Source: CAD feature listing. Evaluate the final solid. Frame: model axes, mm. A direction names the side the tool comes from. Give positions to 0.01 mm unless a question says otherwise; leave off trailing zeros. Order: outer loops, then holes, each group sorted by start corner. A loop starts at its lowest first (then second) coordinate and runs counter-clockwise, first axis right, second up. Notation, with made-up numbers: M 37.5,28 L 67.5,28 A27 cw 67.5,67 Z; hole C 59.25,26 d5. An arc over 180 degrees is marked long. Return JSON: item names as keys, results as strings.
from build123d import *

# Parameters (mm, degrees)
SKETCH1_R               = 10
BOSS_EXTRUDE1_DEPTH     = 3
SKETCH2_R               = 6
BOSS_EXTRUDE2_DEPTH     = 5
TAP_DRILL_FOR_M6_TAP1_D = 5


with BuildPart() as part:
    # Sketch1 → Boss-Extrude1 (new body)
    with BuildSketch(Plane.XY):
        Circle(SKETCH1_R)
    extrude(amount=BOSS_EXTRUDE1_DEPTH)

    # Sketch2 → Boss-Extrude2 (add)
    with BuildSketch(Plane(origin=(0, 0, 0), x_dir=(-1, 0, 0), z_dir=(0, 0, -1))):
        Circle(SKETCH2_R)
    extrude(amount=BOSS_EXTRUDE2_DEPTH)

    # Tap Drill for M6 Tap1 (through all)
    with Locations(Plane(origin=(0, 0, -5), x_dir=(-1, 0, 0), z_dir=(0, 0, -1))):
        with Locations((0, 0)):
            Hole(TAP_DRILL_FOR_M6_TAP1_D / 2)


solid = part.part
1. First-contact query: pin 1 (2 mm diameter, centred on x = 6.5, z = 1, fed in from -Y); pin 2 (2 mm diameter, centred on x = 2, z = 0, fed in from +Y); pin 3 (3 mm diameter, centred on x = 6.5, z = -0.5, fed in from +Y). Flat tips, straight axial feed; report the tip coordinate or a pass-through.
Evaluation:
{"pin 1": "stops at y = -8.35", "pin 2": "stops at y = 9.95", "pin 3": "stops at y = 8.61"}
2. Ray query, probe 1 along Y at (x, z) = (0, -2.5); probe 2 along Z at (x, y) = (7.25, -3.25); probe 3 along Y at (x, z) = (0, 2). Return the intervals inside material, ascending.
Evaluation:
{"probe 1": "y = -6 to -2.5, 2.5 to 6", "probe 2": "z = 0 to 3", "probe 3": "y = -10 to -2.5, 2.5 to 10"}
3. Set-up query: faces 1 (the face through (2, -2, 3)), 2 (the face through (6, 0, -2)). Return all of +Z, -Z, +X, -X, +Y, -Y with unobstructed straight access to the full face (end or side cutting, diameter ignored); none if empty.
Evaluation:
{"face 1": "+Z, +X, -X, +Y, -Y", "face 2": "-Z"}
4. Section query A-A (x = 0). Return loops of the section in (y, z), then the cut area to 3 significant figures.
Evaluation:
{"outline": "M -10,0 L -6,0 L -6,-5 L -2.5,-5 L -2.5,3 L -10,3 Z; M 2.5,-5 L 6,-5 L 6,0 L 10,0 L 10,3 L 2.5,3 Z", "area": "80.0 mm^2"}
5. Draft query along X for faces 3 (the face through (-0.54, -2.44, -0.94)), 4 (the face through (0, -7, 0)), 5 (the face through (-2.17, -9.76, 1.48)). Return one class per face: pulls with the +X half, pulls with the -X half, needs draft (parallel to the pull), parting line crosses it, or undercut.
Evaluation:
{"face 3": "undercut", "face 4": "needs draft", "face 5": "parting line crosses it"}
6. Section query C-C (z = 0.25). Return loops of the section in (x, y).
Evaluation:
{"outline": "C 0,0 d20; hole C 0,0 d5"}
7. Section query D-D (y = 4). Return loops of the section in (x, z), then the cut area to 3 significant figures.
Evaluation:
{"outline": "M -9.17,0 L -4.47,0 L -4.47,-5 L 4.47,-5 L 4.47,0 L 9.17,0 L 9.17,3 L -9.17,3 Z", "area": "99.7 mm^2"}
